Can you work these out from the drawing? Everything is in mm from the part's minimum corner. A direction names the side the tool comes from. Round coordinates to 2 decimals unless told otherwise and drop trailing zeros. Order: outer loops, then holes, each group sorted by start corner. A loop starts at its lowest first (then second) coordinate and runs counter-clockwise, first axis right, second up. Notation, with made-up numbers: (53.5, -27) - (66.5, -27) arc R17 ccw to (66.5, -17) - close; hole circle Ø9 at (3.5, 54). An arc over 180 degrees is marked (long way). Write item = value, one per line.
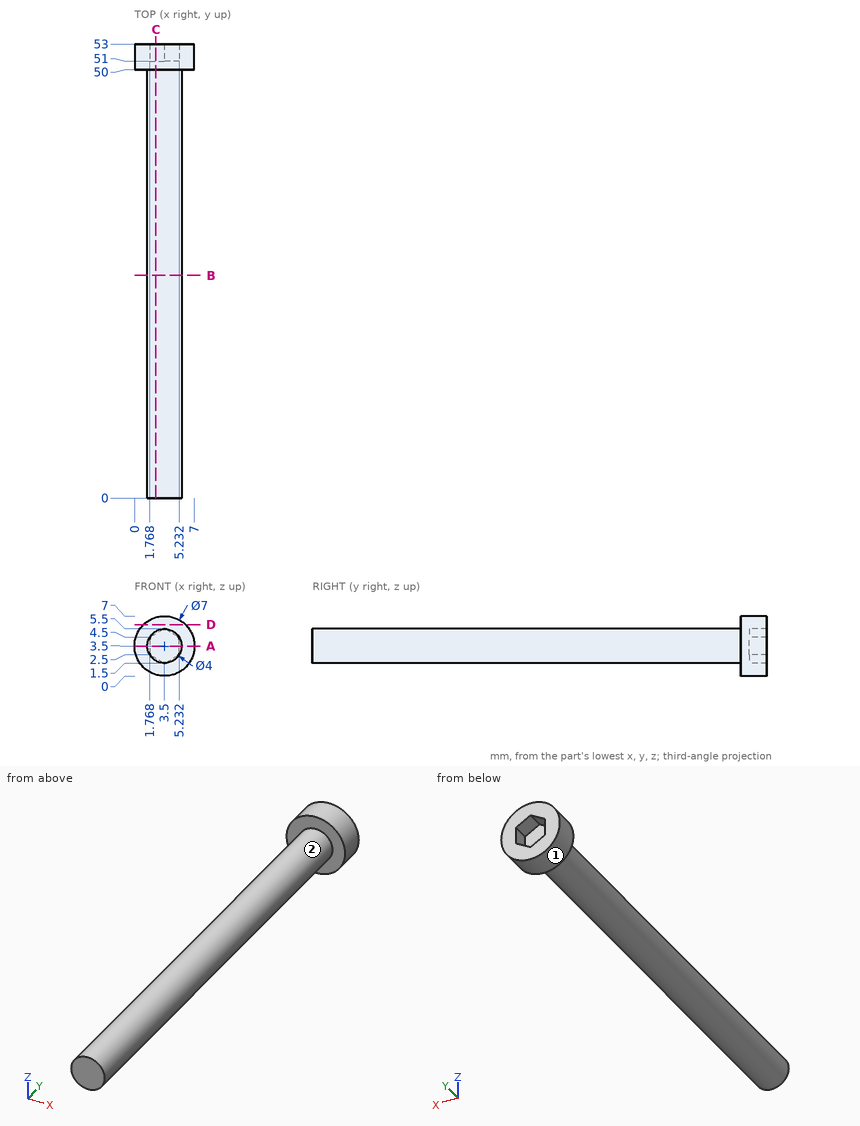
(1) Will these pins go through, and if not, where does the flat tip stop? P1, Ø4, axis at x = 4.5, y = 9.5, coming from the -Z side; P2, Ø1.5, axis at y = 47, z = 4, coming from the -X side; P3, Ø3, axis at y = 24.5, z = 1.5, coming from the +X side.
Computed:
P1 = 1.5
P2 = 1.5
P3 = 5.44
(2) If we section it at C-C (x = 2.5): Write out the boundary of the cut face in (y, z).
Computed:
outline = (0, 1.77) - (50, 1.77) - (50, 0.15) - (53, 0.15) - (53, 2.08) - (51, 2.08) - (51, 4.92) - (53, 4.92) - (53, 6.85) - (50, 6.85) - (50, 5.23) - (0, 5.23) - close
(3) If we section it at D-D (z = 6): Write out the boundary of the cut face in (x, y), plus the area to 3 significant figures.
Computed:
outline = (1.05, 50) - (5.95, 50) - (5.95, 53) - (1.05, 53) - close
area = 14.7 mm^2
(4) If we section it at B-B (y = 26): Write out the boundary of the cut face in (x, z).
Computed:
outline = circle Ø4 at (3.5, 3.5)
(5) If I drill on line 1 (Y direction, x = 1.5, z = 4); line 2 (Y direction, x = 3.25, z = 3.75); line 3 (X direction, y = 13, z = 2.5), over which ranges is the centre line in solid material (lowest first)? Write a range as from..to.
Computed:
line_1 = 50..53
line_2 = 0..51
line_3 = 1.77..5.23
(6) If we section it at A-A (z = 3.5): Write out the boundary of the cut face in (x, y).
Computed:
outline = (0, 50) - (1.5, 50) - (1.5, 0) - (5.5, 0) - (5.5, 50) - (7, 50) - (7, 53) - (5.23, 53) - (5.23, 51) - (1.77, 51) - (1.77, 53) - (0, 53) - close
(7) On a 3-axis mill with a long thin cutter (end or side, diameter ignored), from which of +Z, -Z, +X, -X, +Y, -Y can I reach the whole of each face in a straight line? I mean the marked faces 1 and 2. Say none if no direction works.
Computed:
face_1 = +Y, -Y
face_2 = -Y
